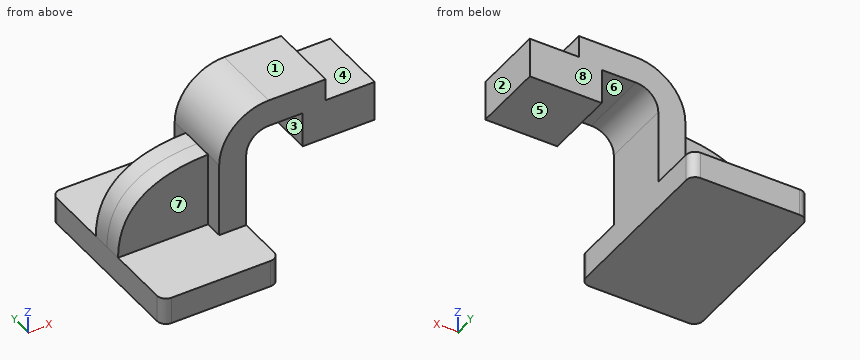
from build123d import *

# Parameters (mm, degrees)
F1_DEPTH = 63.5
F0_W     = 16.2215043542
F0_H     = 3.3740014491
F2_DEPTH = 25.4
F3_DEPTH = 12.7
F4_R     = 6.35


with BuildPart() as f1:
    # F0 (on Front) → F1 (new body, symmetric)
    with BuildSketch(Plane.XZ):
        Polygon((-41.275, -9.525), (41.275, -9.525), (41.275, 9.525), (22.225, 9.525), (-41.275, 9.525), align=None)
    extrude(amount=F1_DEPTH, both=True)

    # F0 (on Front) → F2 (join, symmetric)
    with BuildSketch(Plane.XZ):
        Polygon((97.3541051817, 77.81544), (81.1326008275, 77.81544), (81.1326008275, 52.9319414491), (131.9326008275, 52.9319414491), (131.9326008275, 81.1894414491), (97.3541051817, 81.1894414491), align=None)
        Polygon((-41.275, -9.525), (41.275, -9.525), (41.275, 9.525), (22.225, 9.525), (-41.275, 9.525), align=None)
        with Locations((89.2433530046, 79.5024407246)):
            Rectangle(F0_W, F0_H)
        with BuildLine():
            Line((22.225, 9.525), (41.275, 9.525))
            Line((41.275, 9.525), (41.275, 61.94044))
            ThreePointArc((41.275, 61.94044), (45.9246798487, 73.1657601513), (57.15, 77.81544))
            Line((57.15, 77.81544), (81.1326008275, 77.81544))
            Line((81.1326008275, 77.81544), (81.1326008275, 81.1894414491))
            Line((81.1326008275, 81.1894414491), (97.3541051817, 81.1894414491))
            Line((97.3541051817, 81.1894414491), (97.3541051817, 96.86544))
            Line((97.3541051817, 96.86544), (57.15, 96.86544))
            ThreePointArc((57.15, 96.86544), (32.4542956671, 86.6361443329), (22.225, 61.94044))
            Line((22.225, 61.94044), (22.225, 9.525))
        make_face()
    extrude(amount=F2_DEPTH, both=True)

    # F0 (on Front) → F3 (join, symmetric)
    with BuildSketch(Plane.XZ):
        with BuildLine():
            add(Edge.make_bspline(
                [(-41.275, 9.525), (-41.2206873298, 45.4989261925), (-17.1644557267, 60.9636493027), (22.225, 61.94044)],
                knots=[0, 0, 0, 0, 82.3384985921, 82.3384985921, 82.3384985921, 82.3384985921], degree=3))
            Line((-41.275, 9.525), (22.225, 9.525))
            Line((22.225, 9.525), (22.225, 61.94044))
        make_face()
    extrude(amount=F3_DEPTH, both=True)

    # F4
    f4_edges = [f1.edges().sort_by_distance(p)[0] for p in [
        (41.275, -63.5, 0),
        (-41.275, -63.5, 0),
        (41.275, 63.5, 0),
        (-41.275, 63.5, 0),
    ]]
    fillet(f4_edges, radius=F4_R)


solid = f1.part
Work out the finished part from the listing and answer in its coordinate system (mm). Face numbers are marked on the shaded views. A direction names the side the tool comes from. Round coordinates to 2 decimals unless told otherwise and drop trailing zeros. Loops run counter-clockwise (first coordinate to the right, second up) from the corner with the lowest first, then second, coordinate; pieces in that order, holes last. Notation, with made-up numbers: (74, -32) -> (108, -32) arc R16 cw to (108, -14) -> close; hole circle Ø10 at (-23.75, 3). An arc over 180 degrees is marked (long way). Use one line per item in the form item = value.
(1) Flat-ended cylindrical pins translate along their axes: P1, Ø10.5, axis at x = 107, y = 10.5, coming from the +Z side; P2, Ø3, axis at x = 21.5, z = 46.5, coming from the -Y side; P3, Ø6, axis at x = 10, y = 34.5, coming from the +Z side (3 decimals); P4, Ø8, axis at x = 46.5, y = 40, coming from the -Z side. Find the tip coordinate at first contact, or state that the pin passes through.
Answer list:
P1 = 81.19
P2 = -25.4
P3 = 9.525
P4 = through
(2) Find section D-D on y = 35.5. Give the vertices of the cut face in (x, z) (3 decimals), then the cut area to 3 significant figures.
Answer list:
outline = (-41.275, -9.525) -> (41.275, -9.525) -> (41.275, 9.525) -> (-41.275, 9.525) -> close
area = 1,570 mm2
(3) A tool of negligible diameter and unlimited length cuts with its end or side. For the marked faces 4, 5, 6, 7 and 8, from which of +Z, -Z, +X, -X, +Y, -Y can it reach the whole face along a straight path? Write none if from no direction.
Answer list:
face_4 = +Z, +X, +Y, -Y
face_5 = -Z, +X, +Y, -Y
face_6 = -Z, +Y, -Y
face_7 = +Z, -X, -Y
face_8 = +Z, +X, -X, +Y
(4) For a pull along X with two mould halves and no side action, classify the marked faces 1, 2 and 3 as released by +X, released by -X, zero draft, split by the parting line, or undercut.
Answer list:
face_1 = zero draft
face_2 = released by +X
face_3 = undercut
(5) Straight lines are drawn through the part: line 1 (Z direction, x = 26, y = 33) (3 decimals); line 2 (Y direction, x = 93, z = 61.5); line 3 (Y direction, x = 6, z = 38). For each, find the intervals that lie inside material, in ascending order.
Answer list:
line_1 = -9.525 to 9.525
line_2 = -25.4 to 25.4
line_3 = -12.7 to 12.7
(6) Find section C-C on x = 118. Give the vertices of the cut face in (y, z).
Answer list:
outline = (-25.4, 52.93) -> (25.4, 52.93) -> (25.4, 81.19) -> (-25.4, 81.19) -> close
(7) Find section B-B on z = 3. Give the vertices of the cut face in (x, y) (3 decimals), then the cut area to 3 significant figures.
Answer list:
outline = (-41.275, -57.15) arc R6.35 ccw to (-34.925, -63.5) -> (34.925, -63.5) arc R6.35 ccw to (41.275, -57.15) -> (41.275, 57.15) arc R6.35 ccw to (34.925, 63.5) -> (-34.925, 63.5) arc R6.35 ccw to (-41.275, 57.15) -> close
area = 10,400 mm2
(8) Find section A-A on y = 15.5. Give the vertices of the cut face in (x, z) (3 decimals).
Answer list:
outline = (-41.275, -9.525) -> (41.275, -9.525) -> (41.275, 61.94) arc R15.875 cw to (57.15, 77.815) -> (81.133, 77.815) -> (81.133, 52.932) -> (131.933, 52.932) -> (131.933, 81.189) -> (97.354, 81.189) -> (97.354, 96.865) -> (57.15, 96.865) arc R34.925 ccw to (22.225, 61.94) -> (22.225, 9.525) -> (-41.275, 9.525) -> close
